from build123d import *

# Parameters (mm, degrees)
F1_DEPTH = 4
F3_DEPTH = 27
F5_DEPTH = 3


with BuildPart() as f1:
    # F0 (on Top) → F1 (new body)
    with BuildSketch(Plane.XY):
        Polygon((0, 38.1), (0, 0), (25.4, 0), (25.4, 12.7), (76.2, 12.7), (76.2, 38.1), align=None)
    extrude(amount=F1_DEPTH)

    # F2 (on face) → F3 (join)
    with BuildSketch(Plane.XY.offset(4)):
        Polygon((76.2, 34.1), (76.2, 38.1), (0, 38.1), (0, 0), (4, 0), (4, 34.1), align=None)
    extrude(amount=F3_DEPTH)

    # F4 (on face) → F5 (join)
    with BuildSketch(Plane.XY.offset(31)):
        Polygon((76.2, 26.1), (76.2, 34.1), (4, 34.1), (4, 0), (12, 0), (12, 26.1), align=None)
        Polygon((76.2, 34.1), (76.2, 38.1), (0, 38.1), (0, 0), (4, 0), (4, 34.1), align=None)
    extrude(amount=F5_DEPTH)


solid = f1.part
Design review of the part built by this model. Coordinates are the model's own, in mm. A direction names the side the tool comes from. Give positions to 0.01 mm unless a question says otherwise; leave off trailing zeros. Write each loop counter-clockwise with the first axis right and the second up, starting at its lowest first coordinate (ties: lowest second). Pieces come first, ordered by that corner, then holes. Notation, with made-up numbers: M 87.25,-19 L 126.25,-19 A9 ccw 126.25,-13 Z; hole C 40,11 d2. An arc over 180 degrees is marked long. Answer as a JSON object with one key per item and string values. Group by question number.
1) We need section B-B (y = 28). Give the boundary of the cut face in (x, z).
2) We need section C-C (z = 15). Give the boundary of the cut face in (x, y), and give its area (3 significant figures).
3) Tool access review of faces 4 (the face through (12, 13, 32)), 5 (the face through (76.2, 35, 12)), 6 (the face through (4, 17, 17)), 7 (the face through (50, 12.7, 2)): name each direction out of +Z, -Z, +X, -X, +Y, -Y from which nothing blocks a thin tool from reaching the whole face with its end or side.
4) Mouldability with a two-part tool opening along Z and no side actions: class faces 1 (the face through (40, 21, 4)), 2 (the face through (25.4, 6, 2)), 3 (the face through (38, 24, 0)) as released by +Z, released by -Z, zero draft, split by the parting line, or undercut.
5) Clearance check with flat-ended pins moving along their axes: pin 1 Ø1.2 at (x, z) = (41, 2.5) entering from -Y; pin 2 Ø2.5 at (y, z) = (10, 32) entering from +X; pin 3 Ø3 at (y, z) = (6, 13.5) entering from +X. State where each tip first meets the part, or that it passes through.
6) We need section A-A (x = 8). Give the boundary of the cut face in (y, z), and give its area (3 significant figures).
7) For line 1 along Z through (x, y) = (11.5, 13.5); line 2 along Y through (x, z) = (49, 29); line 3 along X through (y, z) = (14, 18), list the stretches that pass through material, from the lowest coordinate up.
Answer key:
{
 "1": {"outline": "M 0,0 L 76.2,0 L 76.2,4 L 4,4 L 4,31 L 76.2,31 L 76.2,34 L 0,34 Z"},
 "2": {"outline": "M 0,0 L 4,0 L 4,34.1 L 76.2,34.1 L 76.2,38.1 L 0,38.1 Z", "area": "441 mm²"},
 "3": {"face 4": "+Z, +X, -Y", "face 5": "+Z, -Z, +X, +Y, -Y", "face 6": "+X, -Y", "face 7": "+Z, -Z, +X, -Y"},
 "4": {"face 1": "undercut", "face 2": "zero draft", "face 3": "released by -Z"},
 "5": {"pin 1": "stops at y = 12.7", "pin 2": "stops at x = 12", "pin 3": "stops at x = 4"},
 "6": {"outline": "M 0,0 L 38.1,0 L 38.1,34 L 0,34 L 0,31 L 34.1,31 L 34.1,4 L 0,4 Z", "area": "375 mm²"},
 "7": {"line 1": "z = 0 to 4, 31 to 34", "line 2": "y = 34.1 to 38.1", "line 3": "x = 0 to 4"}
}
